Geometry check sheet. Reference: the model listing, model coordinates, mm. A direction names the side the tool comes from. Give positions to 0.01 mm unless a question says otherwise; leave off trailing zeros. Loops run counter-clockwise (first coordinate to the right, second up) from the corner with the lowest first, then second, coordinate; pieces in that order, holes last.
1. Go/stop test with flat-tipped pins: pin 1 Ø4 at (y, z) = (13.5, 8) entering from +X; pin 2 Ø10 at (y, z) = (-6, 15) entering from +X; pin 3 Ø4 at (x, z) = (5, 18) entering from -Y. Record where each tip stops, or that it passes through.
2. Material ranges on L1, parallel to Y at x = 0, z = 15 (3 decimals); L2, parallel to Z at x = -13.5, y = 22; L3, parallel to X at y = 1.5, z = 1.25, recorded low to high.
3. Cross-section at D-D, the plane z = 14.25. Record the cut outline in (x, y) (3 decimals).
4. Release check for a two-part mould opening along Z. For faces 3 (the cylindrical face through (14.246, -22.345, 19.732)), 4 (the flat face through (-22, 10, 18.5)), 5 (the cylindrical face through (-5.2, 23.3, 10.4)), 6 (the flat face through (6, -6, 21)) record: +Z half, -Z half, draft (parallel to the pull), parting line (faces both ways), or undercut.
5. Tool access check on faces 1 (the flat face through (-22, 10, 2.5)), 2 (the flat face through (6, -6, 0)). Record the directions out of +Z, -Z, +X, -X, +Y, -Y that give a thin tool (end or side, any length) a straight path to the whole face; none if there is none.
6. Cross-section at C-C, the plane x = -19. Record the cut outline in (y, z), plus the area to 3 significant figures.
7. Cross-section at A-A, the plane x = 0. Record the cut outline in (y, z) (3 decimals).
Autodesk Inventor part; units mm, degrees
ref_plane "YZ Plane" through (0, 0, 0) normal (1, 0, 0) x (0, 1, 0)
ref_plane "XZ Plane" through (0, 0, 0) normal (0, 1, 0) x (-1, 0, 0)
ref_plane "XY Plane" through (0, 0, 0) normal (0, 0, 1) x (1, 0, 0)
sketch "Sketch1" plane through (0, 0, 0) normal (0, 0, 1) x (1, 0, 0)
  circle A0 centre (0, 0) radius 26.5
  dimension "d0" = 53
extrude "Extrusion1" add sketch "Sketch1" along normal blind 2.5
sketch "Sketch2" plane through (0, 0, 2.5) normal (0, 0, 1) x (1, 0, 0)
  circle A0 centre (0, 0) radius 23.875
  dimension "d3" = 47.75
extrude "Extrusion2" add sketch "Sketch2" along normal blind 16
sketch "Sketch3" plane through (0, 0, 18.5) normal (0, 0, 1) x (1, 0, 0)
  circle A0 centre (0, 0) radius 26.5
  dimension "d6" = 53
extrude "Extrusion3" add sketch "Sketch3" along normal blind 2.5
sketch "Sketch4" plane through (0, 0, 21) normal (0, 0, 1) x (1, 0, 0)
  circle A0 centre (0, 0) radius 7.5
  dimension "d9" = 15
extrude "Extrusion4" cut sketch "Sketch4" against normal blind 30
properties part number "HTD5M 30 Pulley" material "Aluminum 6061"
Result:
1. pin 1: stops at x = 20.92
1. pin 2: stops at x = 26.39
1. pin 3: stops at y = -26.32
2. L1: y = -23.875 to -7.5, 7.5 to 23.875
2. L2: z = 0 to 2.5, 18.5 to 21
2. L3: x = -26.46 to -7.35, 7.35 to 26.46
3. outline: circle Ø47.75 at (0, 0); hole circle Ø15 at (0, 0)
4. face 3: draft
4. face 4: undercut
4. face 5: undercut
4. face 6: +Z half
5. face 1: none
5. face 2: -Z, +X, -X, +Y, -Y
6. outline: (-18.47, 0) - (18.47, 0) - (18.47, 2.5) - (14.46, 2.5) - (14.46, 18.5) - (18.47, 18.5) - (18.47, 21) - (-18.47, 21) - (-18.47, 18.5) - (-14.46, 18.5) - (-14.46, 2.5) - (-18.47, 2.5) - close
6. area: 647 mm2
7. outline: (-26.5, 0) - (-7.5, 0) - (-7.5, 21) - (-26.5, 21) - (-26.5, 18.5) - (-23.875, 18.5) - (-23.875, 2.5) - (-26.5, 2.5) - close; (7.5, 0) - (26.5, 0) - (26.5, 2.5) - (23.875, 2.5) - (23.875, 18.5) - (26.5, 18.5) - (26.5, 21) - (7.5, 21) - close
